Read the model definition and answer for the solid it produces. Units are mm, in the model's axes. Give positions to 0.01 mm unless a question says otherwise; leave off trailing zeros. One line per item, written item: value.
from build123d import *

# Parameters (mm, degrees)
SKETCH1_R           = 2
SKETCH1_R_2         = 5
BOSS_EXTRUDE1_DEPTH = 3
SKETCH2_R           = 8
CUT_EXTRUDE1_DEPTH  = 10
CUT_EXTRUDE2_DEPTH  = 10
FILLET1_R           = 3
FILLET2_R           = 1
FILLET3_R           = 3


with BuildPart() as part:
    # Sketch1 → Boss-Extrude1 (new body)
    with BuildSketch(Plane.XY):
        with BuildLine():
            Line((0, 30), (450, 30))
            ThreePointArc((450, 30), (480, 0), (450, -30))
            Line((450, -30), (0, -30))
            ThreePointArc((0, -30), (-30, 0), (0, 30))
        make_face()
        with Locations((0, 20)):
            Circle(SKETCH1_R, mode=Mode.SUBTRACT)
        with Locations((17.320508076, 10)):
            Circle(SKETCH1_R, mode=Mode.SUBTRACT)
        with Locations((17.320508076, -10)):
            Circle(SKETCH1_R, mode=Mode.SUBTRACT)
        with Locations((0, -20)):
            Circle(SKETCH1_R, mode=Mode.SUBTRACT)
        Circle(SKETCH1_R_2, mode=Mode.SUBTRACT)
        with Locations((-17.320508076, -10)):
            Circle(SKETCH1_R, mode=Mode.SUBTRACT)
        with Locations((-17.320508076, 10)):
            Circle(SKETCH1_R, mode=Mode.SUBTRACT)
    extrude(amount=BOSS_EXTRUDE1_DEPTH)

    # Sketch2 → Cut-Extrude1 (cut)
    with BuildSketch(Plane(origin=(0, 0, 0), x_dir=(-1, 0, 0), z_dir=(0, 0, -1))):
        with Locations((-450, 0)):
            Circle(SKETCH2_R)
    extrude(amount=-CUT_EXTRUDE1_DEPTH, mode=Mode.SUBTRACT)

    # Sketch4 → Cut-Extrude2 (cut)
    with BuildSketch(Plane.XY.offset(3)):
        Polygon((75.051155, 16.751903708), (104.496414244, 16.751903708), (97.010331386, 3.776026753), align=None)
        Polygon((115.236434087, 17.133628969), (159.994947493, 11.590143364), (180.655213039, -0.618195368), (159.994947493, -11.858002091), (118.085145684, -16.966802955), (105.823337098, -0.177570288), align=None)
        Polygon((189.665526052, 18.578346929), (182.941129647, 6.211814834), (165.368544986, 15.767042135), align=None)
        Polygon((199.599828734, 18.578346929), (188.361345274, -0.440625079), (198.44447832, -18.021795356), (236.21688029, -13.651304452), (211.35817569, 15.767042135), align=None)
        Polygon((220.526900823, 17.172694532), (237.960392272, 17.172694532), (260.559362669, 1.057868841), (244.675514904, -10.943884315), align=None)
        Polygon((265.46656767, 6.211814834), (277.833099766, 18.578346929), (248.220353812, 17.874878196), align=None)
        Polygon((165.368544986, -16.358724589), (182.200526719, -6.705265316), (188.690770328, -18.021795356), align=None)
        Polygon((245.637394842, -19.868271823), (269.887796501, -3.220439984), (278.716640894, -18.61460526), align=None)
        Polygon((290.68321902, -21.539751298), (321.940631216, -4.211371592), (335.206376445, -20.70401156), align=None)
        Polygon((341.992933025, 19.183441398), (329.735187473, 1.057868841), (343.614563911, -19.159806148), (373.065049946, 1.057868841), align=None)
        Polygon((273.877820417, 3.11420529), (290.68321902, 20.542728609), (317.209913689, 1.057868841), (284.881711611, -15.886302486), align=None)
        Polygon((305.30736893, 19.270974689), (333.375882047, 18.324324896), (324.94206251, 6.211814834), align=None)
        Polygon((358.198045962, 20.050204211), (388.597492455, 20.050204211), (382.886534474, 8.292807575), align=None)
        Polygon((349.331047186, -24.428108969), (379.030224427, -4.211371592), (391.830023208, -23.92704923), align=None)
        Polygon((386.543005003, -2.048490112), (401.586425759, 20.569577221), (424.881274354, 9.475873595), (434.601030173, -0.440625079), (426.98326683, -8.340846264), (400.664497987, -22.912566492), align=None)
        Polygon((77.908222084, -18.113128875), (99.959146412, -5.986003719), (109.517710051, -19.216558315), align=None)
        Polygon((32.181427401, 14.045195837), (32.181427401, -14.186471438), (52.8225456, -12.955618238), (68.554424875, -10.943884315), (88.302954178, 0), (69.662476286, 10.346921974), (57.571708379, 12.423629667), align=None)
    extrude(amount=-CUT_EXTRUDE2_DEPTH, mode=Mode.SUBTRACT)

    # Fillet1
    # the kernel refuses this fillet: 3 mm, written as the material it adds along each edge
    with BuildSketch(Plane(origin=(32.181427401, 14.045195837, 3), x_dir=(0, -1, 0), z_dir=(0, 0, -1))) as fillet1_piece_1:
        with BuildLine():
            CenterArc((FILLET1_R * 1.06590295895, -FILLET1_R), FILLET1_R, 90, 93.654267812)
            Line((FILLET1_R * 0.0679361503378, -FILLET1_R * 1.06373577423), (0, 0))
            Line((0, 0), (FILLET1_R * 1.06590295895, 0))
        make_face()
    extrude(amount=3)
    with BuildSketch(Plane(origin=(57.571708379, 12.423629667, 3), x_dir=(-0.9979668086083109, 0.06373577422564991, 0), z_dir=(0, 0, -1))) as fillet1_piece_2:
        with BuildLine():
            CenterArc((FILLET1_R * 0.0532106389046, -FILLET1_R), FILLET1_R, 90, 6.091745071)
            Line((-FILLET1_R * 0.0529101714038, -FILLET1_R * 0.00564675611758), (0, 0))
            Line((0, 0), (FILLET1_R * 0.0532106389046, 0))
        make_face()
    extrude(amount=3)
    with BuildSketch(Plane(origin=(69.662476286, 10.346921974, 3), x_dir=(-0.9855678414202016, 0.16928092024302194, 0), z_dir=(0, 0, -1))) as fillet1_piece_3:
        with BuildLine():
            CenterArc((FILLET1_R * 0.169924527084, -FILLET1_R), FILLET1_R, 90, 19.287684891)
            Line((-FILLET1_R * 0.160386998178, -FILLET1_R * 0.0561280297205), (0, 0))
            Line((0, 0), (FILLET1_R * 0.169924527084, 0))
        make_face()
    extrude(amount=3)
    with BuildSketch(Plane(origin=(88.302954178, 0, 3), x_dir=(-0.8743344213622383, 0.48532393266885154, 0), z_dir=(0, 0, -1))) as fillet1_piece_4:
        with BuildLine():
            CenterArc((FILLET1_R * 1.80303637433, -FILLET1_R), FILLET1_R, 90, 121.972748141)
            Line((FILLET1_R * 0.954736326134, -FILLET1_R * 1.52951584323), (0, 0))
            Line((0, 0), (FILLET1_R * 1.80303637433, 0))
        make_face()
    extrude(amount=3)
    with BuildSketch(Plane(origin=(68.554424875, -10.943884315, 3), x_dir=(0.8746742438686059, 0.4847112203290558, 0), z_dir=(0, 0, -1))) as fillet1_piece_5:
        with BuildLine():
            CenterArc((FILLET1_R * 0.191722072286, -FILLET1_R), FILLET1_R, 90, 21.70633324)
            Line((-FILLET1_R * 0.178127385219, -FILLET1_R * 0.0709083044269), (0, 0))
            Line((0, 0), (FILLET1_R * 0.191722072286, 0))
        make_face()
    extrude(amount=3)
    with BuildSketch(Plane(origin=(52.8225456, -12.955618238, 3), x_dir=(0.9919227581955331, 0.1268433749699441, 0), z_dir=(0, 0, -1))) as fillet1_piece_6:
        with BuildLine():
            CenterArc((FILLET1_R * 0.0338255904119, -FILLET1_R), FILLET1_R, 90, 3.874649837)
            Line((-FILLET1_R * 0.0337482743847, -FILLET1_R * 0.00228572587316), (0, 0))
            Line((0, 0), (FILLET1_R * 0.0338255904119, 0))
        make_face()
    extrude(amount=3)
    with BuildSketch(Plane(origin=(32.181427401, -14.186471438, 3), x_dir=(0, 1, 0), z_dir=(0, 0, -1))) as fillet1_piece_7:
        with BuildLine():
            CenterArc((FILLET1_R * 1.06140748795, FILLET1_R), FILLET1_R, 176.587428992, 93.412571008)
            Line((FILLET1_R * 0.0631806961919, FILLET1_R * 1.05952539143), (0, 0))
            Line((0, 0), (FILLET1_R * 1.06140748795, 0))
        make_face()
    extrude(amount=3)

    # Fillet2
    fillet2_edges = [part.edges().sort_by_distance(p)[0] for p in [
        (188.690770328, -18.021795356, 1.5),
        (165.368544986, -16.358724589, 1.5),
        (182.200526719, -6.705265316, 1.5),
        (97.010331386, 3.776026753, 1.5),
        (75.051155, 16.751903708, 1.5),
        (104.496414244, 16.751903708, 1.5),
        (165.368544986, 15.767042135, 1.5),
        (189.665526052, 18.578346929, 1.5),
        (182.941129647, 6.211814834, 1.5),
        (109.517710051, -19.216558315, 1.5),
        (77.908222084, -18.113128875, 1.5),
        (99.959146412, -5.986003719, 1.5),
        (324.94206251, 6.211814834, 1.5),
        (305.30736893, 19.270974689, 1.5),
        (333.375882047, 18.324324896, 1.5),
    ]]
    fillet(fillet2_edges, radius=FILLET2_R)

    # Fillet3
    fillet3_edges = [part.edges().sort_by_distance(p)[0] for p in [
        (244.675514904, -10.943884315, 1.5),
        (220.526900823, 17.172694532, 1.5),
        (237.960392272, 17.172694532, 1.5),
        (260.559362669, 1.057868841, 1.5),
        (199.599828734, 18.578346929, 1.5),
        (211.35817569, 15.767042135, 1.5),
        (236.21688029, -13.651304452, 1.5),
        (198.44447832, -18.021795356, 1.5),
        (188.361345274, -0.440625079, 1.5),
        (400.664497987, -22.912566492, 1.5),
        (386.543005003, -2.048490112, 1.5),
        (401.586425759, 20.569577221, 1.5),
        (424.881274354, 9.475873595, 1.5),
        (434.601030173, -0.440625079, 1.5),
        (426.98326683, -8.340846264, 1.5),
        (341.992933025, 19.183441398, 1.5),
        (373.065049946, 1.057868841, 1.5),
        (343.614563911, -19.159806148, 1.5),
        (329.735187473, 1.057868841, 1.5),
        (284.881711611, -15.886302486, 1.5),
        (273.877820417, 3.11420529, 1.5),
        (290.68321902, 20.542728609, 1.5),
        (317.209913689, 1.057868841, 1.5),
    ]]
    fillet(fillet3_edges, radius=FILLET3_R)


solid = part.part
1) Determine the mould class of faces 1 (the face through (229, 0, 3)), 2 (the face through (479.993, 0.66, 1.479)), 3 (the face through (302.924, 11.552, 1.521)) for opening direction Y: +Y half, -Y half, draft (parallel to the pull), parting line (faces both ways), or undercut.
Reported:
face 1: draft
face 2: parting line
face 3: undercut
2) Each of these flat-tipped pins is pushed along its axis until it touches: pin 1 Ø12 at (x, y) = (169, -2) entering from -Z; pin 2 Ø2.5 at (x, y) = (0, -20) entering from -Z. Where does it stop, or does it pass through?
Reported:
pin 1: stops at z = 0
pin 2: passes through
3) Consider probe 1 along Y at (x, z) = (0, 2.2); probe 2 along Y at (x, z) = (1.5, 1.25); probe 3 along Y at (x, z) = (450, 1.65). Determine where each line is inside the solid, lowest interval first.
Reported:
probe 1: y = -30 to -22, -18 to -5, 5 to 18, 22 to 30
probe 2: y = -30 to -21.32, -18.68 to -4.77, 4.77 to 18.68, 21.32 to 30
probe 3: y = -30 to -8, 8 to 30
